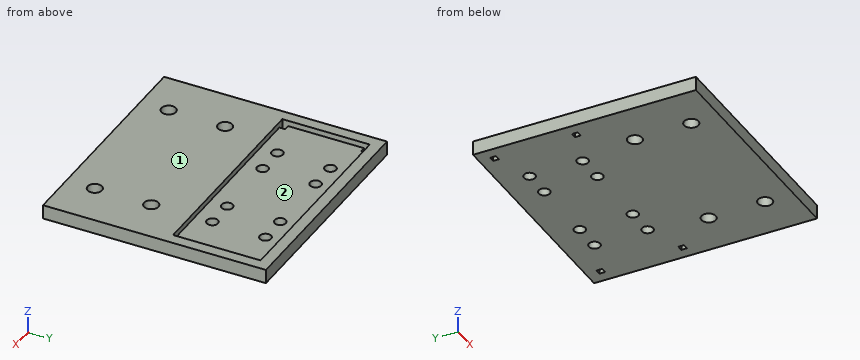
```python
from build123d import *

# Parameters (mm, degrees)
SKETCH1_R           = 2.55
BOSS_EXTRUDE1_DEPTH = 5
SKETCH3_R           = 2.55
SKETCH3_W           = 74
SKETCH3_H           = 31
CUT_EXTRUDE1_DEPTH  = 2
SKETCH4_R           = 2
SKETCH4_W           = 2
SKETCH4_H           = 2
CUT_EXTRUDE2_DEPTH  = 5


with BuildPart() as part:
    # Sketch1 → Boss-Extrude1 (new body)
    with BuildSketch(Plane.XY):
        Polygon((-41, -19.5), (-41, -59.5), (41, -59.5), (41, -19.5), (41, 19.5), (-41, 19.5), align=None)
        with Locations((-25, -29.5)):
            Circle(SKETCH1_R, mode=Mode.SUBTRACT)
        with Locations((-25, -49.5)):
            Circle(SKETCH1_R, mode=Mode.SUBTRACT)
        with Locations((25, -49.5)):
            Circle(SKETCH1_R, mode=Mode.SUBTRACT)
        with Locations((25, -29.5)):
            Circle(SKETCH1_R, mode=Mode.SUBTRACT)
    extrude(amount=BOSS_EXTRUDE1_DEPTH)

    # Sketch3 → Cut-Extrude1 (cut)
    with BuildSketch(Plane.XY.offset(5)):
        with Locations((25, -29.5)):
            Circle(SKETCH3_R)
        with Locations((25, -49.5)):
            Circle(SKETCH3_R)
        with Locations((-25, -49.5)):
            Circle(SKETCH3_R)
        with Locations((-25, -29.5)):
            Circle(SKETCH3_R)
        Rectangle(SKETCH3_W, SKETCH3_H)
    extrude(amount=-CUT_EXTRUDE1_DEPTH, mode=Mode.SUBTRACT)

    # Sketch4 → Cut-Extrude2 (cut)
    with BuildSketch(Plane.XY.offset(3)):
        with Locations((-22, 9.4)):
            Circle(SKETCH4_R)
        with Locations((-12, 9.4)):
            Circle(SKETCH4_R)
        with Locations((12, 9.4)):
            Circle(SKETCH4_R)
        with Locations((22, 9.4)):
            Circle(SKETCH4_R)
        with Locations((22, -9.4)):
            Circle(SKETCH4_R)
        with Locations((12, -9.4)):
            Circle(SKETCH4_R)
        with Locations((-12, -9.4)):
            Circle(SKETCH4_R)
        with Locations((-22, -9.4)):
            Circle(SKETCH4_R)
        with Locations((-36, -14.5)):
            Rectangle(SKETCH4_W, SKETCH4_H)
        with Locations((-36, 14.5)):
            Rectangle(SKETCH4_W, SKETCH4_H)
        with Locations((36, 14.5)):
            Rectangle(SKETCH4_W, SKETCH4_H)
        with Locations((36, -14.5)):
            Rectangle(SKETCH4_W, SKETCH4_H)
    extrude(amount=-CUT_EXTRUDE2_DEPTH, mode=Mode.SUBTRACT)


solid = part.part
```
Here's how the part is built. I have some questions about the finished solid (model axes, mm). Face numbers are marked on the shaded views. Coordinates: 2 decimals unless noted, no trailing zeros. Order: outer loops, then holes, each group sorted by start corner. A loop starts at its lowest first (then second) coordinate and runs counter-clockwise, first axis right, second up.
1) We'd pull the mould along Y, two halves only. Please class the marked faces 1 and 2: +Y half, -Y half, draft (parallel to the pull), parting line (faces both ways), or undercut.
2) Imagine slicing it at A-A on x = -12. List the corners of the cut face in (y, z) for me, and give its area (3 significant figures).
3) Imagine slicing it at D-D on x = 0.5. List the corners of the cut face in (y, z) for me, and give its area (3 significant figures).
4) Imagine slicing it at B-B on y = -49.5. List the corners of the cut face in (x, z) for me.
5) I need wall thicknesses on line 1 (X direction, y = 13.5, z = 3.7); line 2 (Y direction, x = 12, z = 1.5); line 3 (Y direction, x = 25, z = 3.35). Which ranges of each line are inside material? Lowest first, please.
6) Imagine slicing it at C-C on y = 9.4. List the corners of the cut face in (x, z) for me, and give its area (3 significant figures).
7) Will these pins go through, and if not, where does the flat tip stop? pin 1 (5 mm diameter, centred on x = 22, y = 9.4, fed in from +Z); pin 2 (2.5 mm diameter, centred on x = -12, y = 9.4, fed in from -Z).
Response values:
1. face 1: draft
1. face 2: undercut
2. outline: (-59.5, 0) - (-11.4, 0) - (-11.4, 3) - (-15.5, 3) - (-15.5, 5) - (-59.5, 5) - close; (-7.4, 0) - (7.4, 0) - (7.4, 3) - (-7.4, 3) - close; (11.4, 0) - (19.5, 0) - (19.5, 5) - (15.5, 5) - (15.5, 3) - (11.4, 3) - close
2. area: 309 mm2
3. outline: (-59.5, 0) - (19.5, 0) - (19.5, 5) - (15.5, 5) - (15.5, 3) - (-15.5, 3) - (-15.5, 5) - (-59.5, 5) - close
3. area: 333 mm2
4. outline: (-41, 0) - (-27.55, 0) - (-27.55, 5) - (-41, 5) - close; (-22.45, 0) - (22.45, 0) - (22.45, 5) - (-22.45, 5) - close; (27.55, 0) - (41, 0) - (41, 5) - (27.55, 5) - close
5. line 1: x = -41 to -37, 37 to 41
5. line 2: y = -59.5 to -11.4, -7.4 to 7.4, 11.4 to 19.5
5. line 3: y = -59.5 to -52.05, -46.95 to -32.05, -26.95 to -15.5, 15.5 to 19.5
6. outline: (-41, 0) - (-24, 0) - (-24, 3) - (-37, 3) - (-37, 5) - (-41, 5) - close; (-20, 0) - (-14, 0) - (-14, 3) - (-20, 3) - close; (-10, 0) - (10, 0) - (10, 3) - (-10, 3) - close; (14, 0) - (20, 0) - (20, 3) - (14, 3) - close; (24, 0) - (41, 0) - (41, 5) - (37, 5) - (37, 3) - (24, 3) - close
6. area: 214 mm2
7. pin 1: stops at z = 3
7. pin 2: passes through
